Verification items for the finished model (mm, model axes). Coordinates: 2 decimals unless noted, no trailing zeros. Loops run counter-clockwise (first coordinate to the right, second up) from the corner with the lowest first, then second, coordinate; pieces in that order, holes last. Notation, with made-up numbers: (56.25, -5.5) -> (95.25, -5.5) arc R18 cw to (95.25, 6.5) -> close; hole circle Ø10 at (89.25, 54.5). An arc over 180 degrees is marked (long way). Answer as a JSON object with one key per item and string values. Group by question number.
Q1. Gauge pin test, flat ends, axial feed: pin 1 Ø1.5 at (y, z) = (0.5, -1.5) entering from -X; pin 2 Ø0.9 at (x, y) = (-21.5, 1) entering from +Z. Record the tip position at first contact, or that the pin passes through.
Q2. Cross-section at A-A on z = -0.75. Record the boundary of the cut face in (x, y), and give its area (3 significant figures).
Q3. Cross-section at D-D on z = 3.75. Record the boundary of the cut face in (x, y) (3 decimals).
Q4. Cross-section at B-B on y = 1.6. Record the boundary of the cut face in (x, z), and give its area (3 significant figures).
Q5. Scan lines: L1, parallel to X at y = 2.5, z = 2.75 (3 decimals); L2, parallel to X at y = 1.7, z = 6.25 (3 decimals); L3, parallel to X at y = 0.6, z = -0.75. Record each from-to range of solid material in increasing order.
Q6. Cross-section at C-C on x = 3. Record the boundary of the cut face in (y, z), and give its area (3 significant figures).
```python
from build123d import *

# Parameters (mm, degrees)
EXTRUDE_1_DEPTH     = 3
CUT_EXTRUDE_1_DEPTH = 52.230484089
CUT_EXTRUDE_3_DEPTH = 10
FILLET_1_R          = 10


with BuildPart() as part:
    # 草图2 → 凸台-拉伸1 (new body)
    with BuildSketch(Plane(origin=(0, 0, 0), x_dir=(1, 0, 0), z_dir=(0, 1, 0))):
        with BuildLine():
            Line((-12.031587919, -10), (-7.7014609, -7.5))
            ThreePointArc((-7.7014609, -7.5), (10.75, 0), (-7.7014609, 7.5))
            Line((-7.7014609, 7.5), (-12.031587919, 10))
            Line((-12.031587919, 10), (-50, 10))
            Line((-50, 10), (-50, -10))
            Line((-50, -10), (-12.031587919, -10))
        make_face()
    extrude(amount=EXTRUDE_1_DEPTH)

    # 草图3 → 切除-拉伸1 (cut, through all)
    with BuildSketch(Plane(origin=(0, 3, 0), x_dir=(1, 0, 0), z_dir=(0, 1, 0))):
        Polygon((0, 7.071067812), (-7.071067812, 0), (0, -7.071067812), (7.071067812, 0), align=None)
    extrude(amount=-CUT_EXTRUDE_1_DEPTH, mode=Mode.SUBTRACT)

    # 草图5 → 切除-拉伸3 (cut)
    with BuildSketch(Plane(origin=(0, 3, 0), x_dir=(1, 0, 0), z_dir=(0, 1, 0))):
        Polygon((-42, -10), (-42, 0), (-32, 0), (-29, -10), align=None)
    extrude(amount=-CUT_EXTRUDE_3_DEPTH, mode=Mode.SUBTRACT)

    # 圆角1
    # the kernel refuses this fillet: 10 mm, written as the material it takes off along each edge
    with BuildSketch(Plane(origin=(-50, -25, -10), x_dir=(0, 0, 1), z_dir=(0, 1, 0))) as fillet_1_piece_1:
        with BuildLine():
            CenterArc((FILLET_1_R, FILLET_1_R), FILLET_1_R, 180, 90)
            Line((0, FILLET_1_R), (-FILLET_1_R * 0.02, FILLET_1_R))
            Line((-FILLET_1_R * 0.02, FILLET_1_R), (-FILLET_1_R * 0.02, -FILLET_1_R * 0.02))
            Line((-FILLET_1_R * 0.02, -FILLET_1_R * 0.02), (FILLET_1_R, -FILLET_1_R * 0.02))
            Line((FILLET_1_R, -FILLET_1_R * 0.02), (FILLET_1_R, 0))
        make_face()
    extrude(amount=53, mode=Mode.SUBTRACT)
    with BuildSketch(Plane(origin=(-50, -24.494897428, 10), x_dir=(1, 0, 0), z_dir=(0, 1, 0))) as fillet_1_piece_2:
        with BuildLine():
            CenterArc((10, 9.797958971), FILLET_1_R, 180, 78.463040967)
            Line((0, 9.797958971), (-0.2, 9.797958971))
            Line((-0.2, 9.797958971), (-0.2, 0))
            Line((-0.2, 0), (0, -0.2))
            ThreePointArc((0, -0.2), (4, -0.2), (7.96, -0.195959179))
            Line((7.96, -0.195959179), (8, 0))
        make_face()
    extrude(amount=51.989794856, mode=Mode.SUBTRACT)


solid = part.part
```
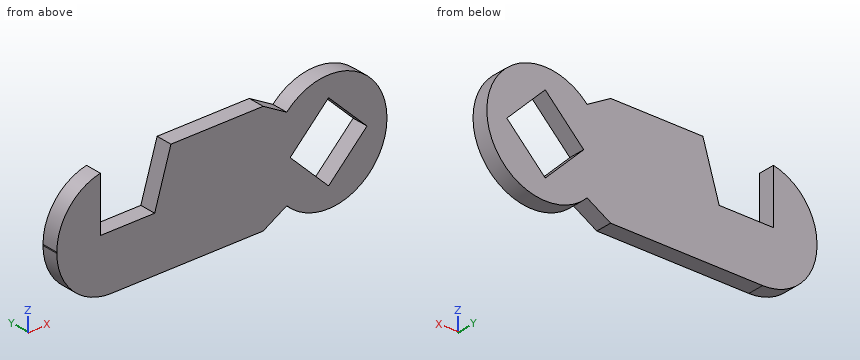
Computed values:
{
 "1": {"pin 1": "stops at x = -49.97", "pin 2": "stops at z = 10"},
 "2": {"outline": "(-49.97, 0) -> (-6.32, 0) -> (-6.32, 3) -> (-49.97, 3) -> close; (6.32, 0) -> (10.72, 0) -> (10.72, 3) -> (6.32, 3) -> close", "area": "144 mm²"},
 "3": {"outline": "(-49.349, 0) -> (-42, 0) -> (-42, 3) -> (-49.349, 3) -> close; (-30.875, 0) -> (-3.321, 0) -> (-3.321, 3) -> (-30.875, 3) -> close; (3.321, 0) -> (10.075, 0) -> (10.075, 3) -> (3.321, 3) -> close"},
 "4": {"outline": "(-50, 0) arc R10 ccw to (-40, -10) -> (-12.03, -10) -> (-7.7, -7.5) arc R10.75 ccw (long way) to (-7.7, 7.5) -> (-12.03, 10) -> (-29, 10) -> (-32, 0) -> (-42, 0) -> (-42, 10) arc R10 ccw to (-50, 0.2) -> close; hole (-7.07, 0) -> (0, -7.07) -> (7.07, 0) -> (0, 7.07) -> close", "area": "911 mm²"},
 "5": {"L1": "x = -49.67 to -42, -31.175 to -4.321, 4.321 to 10.392", "L2": "x = -47.964 to -42, -30.125 to -0.821, 0.821 to 8.746", "L3": "x = -49.97 to -6.32, 6.32 to 10.72"},
 "6": {"outline": "(0, -10.32) -> (3, -10.32) -> (3, -4.07) -> (0, -4.07) -> close; (0, 4.07) -> (3, 4.07) -> (3, 10.32) -> (0, 10.32) -> close", "area": "37.5 mm²"}
}
